```python
from build123d import *

# Parameters (mm, degrees)
F0_W      = 11
F0_H      = 15
F1_DEPTH  = 1
F3_DEPTH  = 0.35
F5_DEPTH  = 0.65
F6_R      = 0.2
F7_R      = 0.4
F8_R      = 0.2
F9_R      = 0.4
F11_DEPTH = 9.7
F12_R     = 0.8


with BuildPart() as f1:
    # F0 (on Top) → F1 (new body)
    with BuildSketch(Plane.XY):
        with Locations((5.5, 7.5)):
            Rectangle(F0_W, F0_H)
    extrude(amount=F1_DEPTH)

    # F2 (on face) → F3 (cut)
    with BuildSketch(Plane.XY.offset(1)):
        with BuildLine():
            Line((0, 14.0084757939), (0, 0))
            Line((0, 0), (11, 0))
            Line((11, 0), (11, 14.0084757939))
            ThreePointArc((11, 14.0084757939), (5.5, 13.5), (0, 14.0084757939))
        make_face()
    extrude(amount=-F3_DEPTH, mode=Mode.SUBTRACT)

    # F4 (on face) → F5 (cut, through all)
    with BuildSketch(Plane.XY.offset(0.65)):
        Polygon((0, 0), (1.3, 0), (1.3, 5.1), (0, 6.4), align=None)
        Polygon((0, 9.4313708499), (0, 7.5313708499), (0.7, 7.5313708499), (0.7, 8.7313708499), align=None)
    extrude(amount=-F5_DEPTH, mode=Mode.SUBTRACT)

    # F6
    f6_edges = [f1.edges().sort_by_distance(p)[0] for p in [
        (0.7, 7.531371, 0.325),
    ]]
    fillet(f6_edges, radius=F6_R)

    # F7
    f7_edges = [f1.edges().sort_by_distance(p)[0] for p in [
        (0.7, 8.731371, 0.325),
    ]]
    fillet(f7_edges, radius=F7_R)

    # F8
    f8_edges = [f1.edges().sort_by_distance(p)[0] for p in [
        (5.5, 13.5, 0.65),
    ]]
    fillet(f8_edges, radius=F8_R)

    # F9
    f9_edges = [f1.edges().sort_by_distance(p)[0] for p in [
        (1.3, 5.1, 0.325),
    ]]
    fillet(f9_edges, radius=F9_R)

    # F10 (on face) → F11 (cut, through all)
    with BuildSketch(Plane.YZ.offset(11)):
        Polygon((0.52, 0), (0, 0.3), (0, 0), align=None)
    extrude(amount=-F11_DEPTH, mode=Mode.SUBTRACT)

    # F12
    f12_edges = [f1.edges().sort_by_distance(p)[0] for p in [
        (11, 0, 0.475),
        (1.3, 0, 0.475),
        (0, 15, 0.5),
        (11, 15, 0.5),
    ]]
    fillet(f12_edges, radius=F12_R)


solid = f1.part
```
Here's how the part is built. I have some questions about the finished solid (model axes, mm). Coordinates: 2 decimals unless noted, no trailing zeros. Order: outer loops, then holes, each group sorted by start corner. A loop starts at its lowest first (then second) coordinate and runs counter-clockwise, first axis right, second up.
Item 1: I'm going to push flat-ended pins straight in: pin 1 Ø0.5 at (y, z) = (8, 0.5) entering from -X; pin 2 Ø3.5 at (x, y) = (7, 7) entering from +Z. Where does each tip first touch, or does it pass through?
Response values:
pin 1: stops at x = 0.7
pin 2: stops at z = 0.65
Item 2: If we section it at B-B, the plane z = 0.15: List the corners of the cut face in (x, y) for me.
Response values:
outline: (0, 6.4) - (1.18, 5.22) arc R0.4 cw to (1.3, 4.93) - (1.3, 0.8) arc R0.8 ccw to (1.51, 0.26) - (10.79, 0.26) arc R0.8 ccw to (11, 0.8) - (11, 14.2) arc R0.8 ccw to (10.2, 15) - (0.8, 15) arc R0.8 ccw to (0, 14.2) - (0, 9.43) - (0.58, 8.85) arc R0.4 cw to (0.7, 8.57) - (0.7, 7.73) arc R0.2 cw to (0.5, 7.53) - (0, 7.53) - close
Item 3: I need wall thicknesses on probe 1 along Z at (x, y) = (10.5, 1.25); probe 2 along X at (y, z) = (4.25, 0.35). Which ranges of each line are inside material? Lowest first, please.
Response values:
probe 1: z = 0 to 0.65
probe 2: x = 1.3 to 11
Item 4: If we section it at A-A, the plane y = 2.5: List the corners of the cut face in (x, z) for me, then the cut area to 4 significant figures.
Response values:
outline: (1.3, 0) - (11, 0) - (11, 0.65) - (1.3, 0.65) - close
area: 6.305 mm2
Item 5: If we section it at C-C, the plane y = 11: List the corners of the cut face in (x, z) for me, then the cut area to 3 significant figures.
Response values:
outline: (0, 0) - (11, 0) - (11, 0.65) - (0, 0.65) - close
area: 7.15 mm2
